from build123d import *

# Parameters (mm, degrees)
BOSS_EXTRUDE1_DEPTH = 28
BOSS_EXTRUDE5_DEPTH = 5
BOSS_EXTRUDE6_DEPTH = 10
BOSS_EXTRUDE7_REACH = 204.915
BOSS_EXTRUDE8_START = 15
BOSS_EXTRUDE8_DEPTH = 15


with BuildPart() as part:
    # Sketch3 → Boss-Extrude1 (new body)
    with BuildSketch(Plane.XY):
        with BuildLine():
            Line((10.849101299, -10.749101299), (10.849101299, -4.6))
            Line((10.849101299, -4.6), (12.849101299, -2.6))
            Line((12.849101299, -2.6), (38.011182565, -2.6))
            ThreePointArc((38.011182565, -2.6), (4.13933396, -37.874475764), (-36.552247828, -10.749101299))
            Line((-36.552247828, -10.749101299), (-38.1, -10.749101299))
            Line((-38.1, -10.749101299), (-38.1, 10.749101299))
            Line((-38.1, 10.749101299), (-36.552247828, 10.749101299))
            ThreePointArc((-36.552247828, 10.749101299), (4.13933396, 37.874475764), (38.011182565, 2.6))
            Line((38.011182565, 2.6), (12.849101299, 2.6))
            Line((12.849101299, 2.6), (10.849101299, 4.6))
            Line((10.849101299, 4.6), (10.849101299, 10.749101299))
            Line((10.849101299, 10.749101299), (-30.849101299, 10.749101299))
            Line((-30.849101299, 10.749101299), (-30.849101299, -10.749101299))
            Line((-30.849101299, -10.749101299), (10.849101299, -10.749101299))
        make_face()
    extrude(amount=-BOSS_EXTRUDE1_DEPTH)

    # Sketch7 → Boss-Extrude5 (add)
    with BuildSketch(Plane(origin=(0, 0, -28), x_dir=(-1, 0, 0), z_dir=(0, 0, -1))):
        with BuildLine():
            Line((-12.849101299, 2.6), (-12.849101299, -2.6))
            Line((-12.849101299, -2.6), (-38.011182565, -2.6))
            ThreePointArc((-38.011182565, -2.6), (-4.13933396, -37.874475764), (36.552247828, -10.749101299))
            Line((36.552247828, -10.749101299), (38.1, -10.749101299))
            Line((38.1, -10.749101299), (38.1, 10.749101299))
            Line((38.1, 10.749101299), (36.552247828, 10.749101299))
            ThreePointArc((36.552247828, 10.749101299), (-4.13933396, 37.874475764), (-38.011182565, 2.6))
            Line((-38.011182565, 2.6), (-12.849101299, 2.6))
        make_face()
    extrude(amount=BOSS_EXTRUDE5_DEPTH)

    # Sketch8 → Boss-Extrude6 (add, symmetric)
    with BuildSketch(Plane(origin=(0, 0, 0), x_dir=(1, 0, 0), z_dir=(0, 1, 0))):
        Polygon((-3.957864376, 33), (102.108152802, 139.066017178), (95.03708499, 146.13708499), (-18.1, 33), align=None)
    extrude(amount=BOSS_EXTRUDE6_DEPTH, both=True)

    # Boss-Extrude7: up to this plane
    boss_extrude7_end = Plane(origin=(0, 0, -33), z_dir=(0, 0, -1))
    # Sketch9 → Boss-Extrude7 (add, up to the surface)
    with BuildSketch(Plane(origin=(120.58708499, 0, -120.58708499), x_dir=(-0.70710678118655, 0, -0.7071067811865451), z_dir=(0.7071067811865451, 0, -0.70710678118655)), mode=Mode.PRIVATE) as boss_extrude7_sk1:
        Polygon((26.133156519, 5), (21.133156519, 5), (21.133156519, 10), (16.133156519, 10), (16.133156519, -10), (21.133156519, -10), (21.133156519, -5), (26.133156519, -5), align=None)
    boss_extrude7_tool1 = split(extrude(boss_extrude7_sk1.sketch, amount=-BOSS_EXTRUDE7_REACH, mode=Mode.PRIVATE), bisect_by=boss_extrude7_end, keep=Keep.BOTH, mode=Mode.PRIVATE)
    add(boss_extrude7_tool1.solids().sort_by_distance((106.232942, 0, -134.941228))[0])

    # Sketch12 → Boss-Extrude8 (add)
    with BuildSketch(Plane.XY.offset(BOSS_EXTRUDE8_START)):
        with BuildLine():
            Line((-36.552247828, 10.749101299), (18.5, 10.749101299))
            Line((18.5, 10.749101299), (18.5, 2.6))
            Line((18.5, 2.6), (38.011182565, 2.6))
            ThreePointArc((38.011182565, 2.6), (4.13933396, 37.874475764), (-36.552247828, 10.749101299))
        make_face()
        with BuildLine():
            Line((-36.552247828, -10.749101299), (18.5, -10.749101299))
            Line((18.5, -10.749101299), (18.5, -2.6))
            Line((18.5, -2.6), (38.011182565, -2.6))
            ThreePointArc((38.011182565, -2.6), (4.13933396, -37.874475764), (-36.552247828, -10.749101299))
        make_face()
    extrude(amount=-BOSS_EXTRUDE8_DEPTH)


solid = part.part
Design review of the part built by this model. Coordinates are the model's own, in mm. A direction names the side the tool comes from. Round coordinates to 2 decimals unless told otherwise and drop trailing zeros. Write each loop counter-clockwise with the first axis right and the second up, starting at its lowest first coordinate (ties: lowest second). Pieces come first, ordered by that corner, then holes. Notation, with made-up numbers: (-28.75, 66.5) - (-19.75, 66.5) arc R21 ccw to (-19.75, 103.5) - close; hole circle Ø5 at (9, 21). An arc over 180 degrees is marked (long way). Use a Markdown table: item, result. Add a question column.
1. For faces 4 (the face through (-9, 0, -28)), 5 (the face through (18.5, 7, 8)), 6 (the face through (57, -10, -83)), 7 (the face through (52, 5, -85)), 8 (the face through (12.849, 0, -30)), list the 3-axis set-ups (+Z, -Z, +X, -X, +Y, -Y) from which the entire face can be reached by the end or side of a thin tool; tool diameter is ignored.
2. Clearance check with flat-ended pins moving along their axes: pin 1 (2 mm diameter, centred on x = 83.5, y = 2, fed in from -Z); pin 2 (0.8 mm diameter, centred on x = -37, z = -24, fed in from -Y); pin 3 (4 mm diameter, centred on y = 0.5, z = -30.5, fed in from +X). State where each tip first meets the part, or that it passes through.
3. Mouldability with a two-part tool opening along X and no side actions: class faces 1 (the face through (0, 21, 15)), 2 (the face through (4.877, -37.787, -8.664)), 3 (the face through (-9, 10.749, -6)) as +X half, -X half, draft (parallel to the pull), parting line (faces both ways), or undercut.
4. We need section D-D (x = -22.5). State the section outline as (y, z) points.
5. We need section C-C (y = 7). State the section outline as (x, z) points.
6. We need section A-A (x = 15). State the section outline as (y, z) points.
7. Wall thickness on probe 1 along Z at (x, y) = (31, -3); probe 2 along X at (y, z) = (5.5, -105); probe 3 along Z at (x, y) = (0.5, -35): over which ranges is each line inside the solid? List them lowest first.
8. We need section B-B (z = -19.5). State the section outline as (x, y) points.
Output:
| question | item | result |
|---|---|---|
| 1 | face 4 | +Z |
| 1 | face 5 | +Z, -X |
| 1 | face 6 | -Z, +X, -X, -Y |
| 1 | face 7 | +Y |
| 1 | face 8 | +Z, +X |
| 2 | pin 1 | stops at z = -135.6 |
| 2 | pin 2 | stops at y = -10.75 |
| 2 | pin 3 | stops at x = 12.85 |
| 3 | face 1 | draft |
| 3 | face 2 | parting line |
| 3 | face 3 | undercut |
| 4 | outline | (-30.75, -33) - (30.75, -33) - (30.75, 15) - (10.75, 15) - (10.75, -28) - (-10.75, -28) - (-10.75, 15) - (-30.75, 15) - close |
| 5 | outline | (-38.1, -33) - (-18.1, -33) - (95.04, -146.14) - (102.11, -139.07) - (-3.96, -33) - (3.11, -33) - (105.64, -135.53) - (109.18, -131.99) - (10.18, -33) - (37.45, -33) - (37.45, 15) - (18.5, 15) - (18.5, 0) - (10.85, 0) - (10.85, -28) - (-30.85, -28) - (-30.85, 0) - (-38.1, 0) - close |
| 6 | outline | (-35.02, -33) - (-2.6, -33) - (-2.6, 0) - (-10.75, 0) - (-10.75, 15) - (-35.02, 15) - close; (-10, -66.1) - (10, -66.1) - (10, -51.96) - (5, -51.96) - (5, -44.89) - (10, -44.89) - (10, -37.82) - (-10, -37.82) - (-10, -44.89) - (-5, -44.89) - (-5, -51.96) - (-10, -51.96) - close; (2.6, -33) - (35.02, -33) - (35.02, 15) - (10.75, 15) - (10.75, 0) - (2.6, 0) - close |
| 7 | probe 1 | z = -82.1 to -53.82, -33 to 15 |
| 7 | probe 2 | x = 53.9 to 68.04, 75.11 to 82.18 |
| 7 | probe 3 | z = -33 to 15 |
| 8 | outline | (-38.1, -10.75) - (-36.55, -10.75) arc R38.1 ccw to (38.01, -2.6) - (12.85, -2.6) - (10.85, -4.6) - (10.85, -10.75) - (-30.85, -10.75) - (-30.85, 10.75) - (10.85, 10.75) - (10.85, 4.6) - (12.85, 2.6) - (38.01, 2.6) arc R38.1 ccw to (-36.55, 10.75) - (-38.1, 10.75) - close |
